Geometry check sheet. Reference: the model listing, model coordinates, mm. A direction names the side the tool comes from. Coordinates: 2 decimals unless noted, no trailing zeros. Write each loop counter-clockwise with the first axis right and the second up, starting at its lowest first coordinate (ties: lowest second). Pieces come first, ordered by that corner, then holes. Notation, with made-up numbers: (31, -1.75) -> (58, -1.75) arc R25 ccw to (58, 12.25) -> close; hole circle Ø1 at (36, 44). An arc over 180 degrees is marked (long way). Answer in a Markdown table with one row per item. Add a question column.
Q1. Thickness scan on line 1 (X direction, y = 1, z = -30); line 2 (Z direction, x = -25.5, y = -10.5); line 3 (Z direction, x = -24.5, y = -5). Record the ranges inside material, lowest first.
Q2. Gauge pin test, flat ends, axial feed: P1, Ø12, axis at y = 1, z = 57.5, coming from the -X side; P2, Ø10, axis at x = -19, y = -23.5, coming from the +Z side; P3, Ø12, axis at x = -23, z = 60.5, coming from the -Y side; P4, Ø3, axis at y = -23, z = 91, coming from the -X side. Record the tip position at first contact, or that the pin passes through.
Q3. Release check for a two-part mould opening along Z. For faces 4 (the face through (0, 0, -71.12)), 5 (the face through (-12.434, -3.916, 26.924)), 6 (the face through (2.645, -20.147, 91.896)) record: pulls with the +Z half, pulls with the -Z half, needs draft (parallel to the pull), parting line crosses it, or undercut.
Q4. Section check C-C, the plane z = 0.5. Record the boundary of the cut face in (x, y).
Q5. Section check D-D, the plane z = 80. Record the boundary of the cut face in (x, y).
Q6. Tool access check on faces 1 (the face through (6.12, 27.57, 2.16)), 2 (the face through (6.39, 28.76, -47.39)), 3 (the face through (4.714, 21.231, -18.768)). Record the directions out of +Z, -Z, +X, -X, +Y, -Y that give a thin tool (end or side, any length) a straight path to the whole face; none if there is none.
Q7. Section check A-A, the plane y = 0. Record the boundary of the cut face in (x, z).
```python
from build123d import *

# Parameters (mm, degrees)
F2_DEPTH = 104.11185
F3_DEPTH = 25.4


with BuildPart() as f1:
    # F0 (on Front) → F1 (revolve)
    with BuildSketch(Plane.XZ):
        with BuildLine():
            Line((0, -45.72), (0, 0))
            Line((0, 0), (0, 45.72))
            Line((0, 45.72), (-20.32, 45.72))
            Line((-20.32, 45.72), (-20.32, 35.56))
            ThreePointArc((-20.32, 35.56), (-15.1165623924, 33.8078630493), (-13.0358416779, 28.7268839961))
            Line((-13.0358416779, 28.7268839961), (-13.0358416779, 25.1708839961))
            ThreePointArc((-13.0358416779, 25.1708839961), (-11.6763486852, 21.8887775753), (-8.3942422643, 20.5292845826))
            ThreePointArc((-8.3942422643, 20.5292845826), (-5.5456340699, 19.1163985733), (-4.9467060106, 15.9935632109))
            ThreePointArc((-4.9467060106, 15.9935632109), (-7.3062957159, 10.2970097428), (-13.002849184, 7.9374200376))
            Line((-13.002849184, 7.9374200376), (-28.242849184, 7.9374200376))
            Line((-28.242849184, 7.9374200376), (-28.242849184, -3.4583220258))
            Line((-28.242849184, -3.4583220258), (-21.2328514445, -3.4583220258))
            Line((-21.2328514445, -3.4583220258), (-21.2328514445, -18.3975605232))
            Line((-21.2328514445, -18.3975605232), (-29.4625001389, -24.3229104143))
            Line((-29.4625001389, -24.3229104143), (-29.4625001389, -45.72))
            Line((-29.4625001389, -45.72), (0, -45.72))
        make_face()
    revolve(axis=Axis((0, 0, 22.86), (0, 0, 1)))

    # F2 (add): a face of the model
    f2_faces = [f1.faces().sort_by_distance(p)[0] for p in [
        (0, 0, 45.72),
    ]]
    extrude(f2_faces, amount=F2_DEPTH)

    # F3 (add): a face of the model
    f3_faces = [f1.faces().sort_by_distance(p)[0] for p in [
        (0, 0, -45.72),
    ]]
    extrude(f3_faces, amount=F3_DEPTH)


solid = f1.part
```
Calculated:
| question | item | result |
|---|---|---|
| 1 | line 1 | x = -29.45 to 29.45 |
| 1 | line 2 | z = -71.12 to -22.97, -3.46 to 7.94 |
| 1 | line 3 | z = -71.12 to -21.11, -3.46 to 7.94 |
| 2 | P1 | stops at x = -20.32 |
| 2 | P2 | stops at z = 7.94 |
| 2 | P3 | stops at y = -11.13 |
| 2 | P4 | passes through |
| 3 | face 4 | pulls with the -Z half |
| 3 | face 5 | undercut |
| 3 | face 6 | needs draft |
| 4 | outline | circle Ø56.49 at (0, 0) |
| 5 | outline | circle Ø40.64 at (0, 0) |
| 6 | face 1 | +Z |
| 6 | face 2 | +Z, -Z |
| 6 | face 3 | none |
| 7 | outline | (-29.46, -71.12) -> (29.46, -71.12) -> (29.46, -24.32) -> (21.23, -18.4) -> (21.23, -3.46) -> (28.24, -3.46) -> (28.24, 7.94) -> (13, 7.94) arc R8.06 cw to (4.95, 15.99) arc R3.58 cw to (8.39, 20.53) arc R4.64 ccw to (13.04, 25.17) -> (13.04, 28.73) arc R6.6 cw to (20.32, 35.56) -> (20.32, 149.83) -> (-20.32, 149.83) -> (-20.32, 35.56) arc R6.6 cw to (-13.04, 28.73) -> (-13.04, 25.17) arc R4.64 ccw to (-8.39, 20.53) arc R3.58 cw to (-4.95, 15.99) arc R8.06 cw to (-13, 7.94) -> (-28.24, 7.94) -> (-28.24, -3.46) -> (-21.23, -3.46) -> (-21.23, -18.4) -> (-29.46, -24.32) -> close |
